The model under review builds one solid part; all positions refer to its coordinate system, in mm. A direction names the side the tool comes from. Coordinates: 2 decimals unless noted, no trailing zeros. Order: outer loops, then holes, each group sorted by start corner. A loop starts at its lowest first (then second) coordinate and runs counter-clockwise, first axis right, second up. Notation, with made-up numbers: (6, -34) - (18, -34) arc R30 ccw to (18, -12) - close; hole circle Ø2 at (73.5, -22). An arc over 180 degrees is marked (long way). Answer in a Markdown table with one row per item.
```python
from build123d import *

# Parameters (mm, degrees)
BOSS_EXTRUDE1_DEPTH = 40
SKETCH3_OUTSIDE_W   = 68.248
SKETCH3_OUTSIDE_H   = 58.248
CUT_EXTRUDE1_DEPTH  = 40
SKETCH4_OUTSIDE_W   = 68.248
SKETCH4_OUTSIDE_H   = 58.248
SKETCH4_OUTSIDE_R   = 10
CUT_EXTRUDE4_DEPTH  = 40


with BuildPart() as part:
    # Sketch2 → Boss-Extrude1 (new body)
    with BuildSketch(Plane.XY):
        with BuildLine():
            Line((2.466960352, 28.854625551), (-27.533039648, 28.854625551))
            Line((-27.533039648, 28.854625551), (-27.533039648, -1.145374449))
            ThreePointArc((-27.533039648, -1.145374449), (-21.675175271, -15.287510073), (-7.533039648, -21.145374449))
            Line((-7.533039648, -21.145374449), (22.466960352, -21.145374449))
            Line((22.466960352, -21.145374449), (22.466960352, -11.145374449))
            Line((22.466960352, -11.145374449), (-7.533039648, -11.145374449))
            ThreePointArc((-7.533039648, -11.145374449), (-14.604107459, -8.216442261), (-17.533039648, -1.145374449))
            Line((-17.533039648, -1.145374449), (-17.533039648, 18.854625551))
            Line((-17.533039648, 18.854625551), (2.466960352, 18.854625551))
            Line((2.466960352, 18.854625551), (2.466960352, 28.854625551))
        make_face()
    extrude(amount=BOSS_EXTRUDE1_DEPTH)

    # Sketch3 outside → Cut-Extrude1 (cut)
    with BuildSketch(Plane(origin=(0, 28.854625551, 0), x_dir=(1, 0, 0), z_dir=(0, 1, 0))):
        with Locations((-2.533, -20)):
            Rectangle(SKETCH3_OUTSIDE_W, SKETCH3_OUTSIDE_H)
        with BuildLine():
            Line((-27.533039648, 0), (-27.533039648, -40))
            Line((-27.533039648, -40), (-7.533039648, -40))
            ThreePointArc((-7.533039648, -40), (-0.461971836, -37.071067812), (2.466960352, -30))
            Line((2.466960352, -30), (2.466960352, -10))
            ThreePointArc((2.466960352, -10), (-0.461971836, -2.928932188), (-7.533039648, 0))
            Line((-7.533039648, 0), (-27.533039648, 0))
        make_face(mode=Mode.SUBTRACT)
    extrude(amount=-CUT_EXTRUDE1_DEPTH, mode=Mode.SUBTRACT)

    # Sketch4 outside → Cut-Extrude4 (cut)
    # profile 1 of 2: a face of its own
    with BuildSketch(Plane.XZ.offset(21.145374449)):
        with Locations((-2.533, 20)):
            Rectangle(SKETCH4_OUTSIDE_W, SKETCH4_OUTSIDE_H)
        with BuildLine():
            Line((-7.533039648, 40), (-27.533039648, 40))
            Line((-27.533039648, 40), (-27.533039648, 0))
            Line((-27.533039648, 0), (-7.533039648, 0))
            Line((-7.533039648, 0), (2.466960352, 0))
            ThreePointArc((2.466960352, 0), (22.466960352, 20), (2.466960352, 40))
            Line((2.466960352, 40), (-7.533039648, 40))
        make_face(mode=Mode.SUBTRACT)
    # profile 2 of 2: a face of its own
    with BuildSketch(Plane.XZ.offset(21.145374449)):
        with Locations(Location((2.466960352, 20, 0), (0, 0, 180))):
            Circle(SKETCH4_OUTSIDE_R)
    extrude(amount=-CUT_EXTRUDE4_DEPTH, mode=Mode.SUBTRACT)


solid = part.part
```
Item 1: We need section A-A, the plane x = 10. Write out the cut boundary in (y, z).
Check values:
| item | result |
|---|---|
| outline | (-21.15, 1.47) - (-11.15, 1.47) - (-11.15, 13.42) - (-21.15, 13.42) - close; (-21.15, 26.58) - (-11.15, 26.58) - (-11.15, 38.53) - (-21.15, 38.53) - close |
Item 2: To check wall thickness, follow line 1 (X direction, y = -13.5, z = 20); line 2 (X direction, y = -19, z = 20); line 3 (X direction, y = 7.5, z = 38). State the ranges of each line that lie inside material, in increasing order. Write a range as from..to.
Check values:
| item | result |
|---|---|
| line 1 | -23.26..-7.53, 12.47..22.47 |
| line 2 | -16.54..-7.53, 12.47..22.47 |
| line 3 | -27.53..-17.53 |
Item 3: Mouldability with a two-part tool opening along Y and no side actions: class faces 5 (the face through (-8, 18.855, 20)), 6 (the face through (-0.54, 23.92, 37.15)), 7 (the face through (-21.83, -15.13, 19.72)) as +Y half, -Y half, draft (parallel to the pull), parting line (faces both ways), or undercut.
Check values:
| item | result |
|---|---|
| face 5 | undercut |
| face 6 | draft |
| face 7 | -Y half |
Item 4: We need section B-B, the plane z = 15.5. Write out the cut boundary in (x, y), then the cut area to 3 significant figures.
Check values:
| item | result |
|---|---|
| outline | (-27.53, -1.15) arc R20 ccw to (-7.53, -21.15) - (-6.46, -21.15) - (-6.46, -11.15) - (-7.53, -11.15) arc R10 cw to (-17.53, -1.15) - (-17.53, 18.85) - (2.47, 18.85) - (2.47, 28.85) - (-27.53, 28.85) - close; (11.4, -21.15) - (21.95, -21.15) - (21.95, -11.15) - (11.4, -11.15) - close |
| area | 852 mm^2 |
Item 5: Clearance check with flat-ended pins moving along their axes: pin 1 Ø4 at (y, z) = (-5, 26) entering from -X; pin 2 Ø8 at (y, z) = (2, 34.5) entering from +X; pin 3 Ø12 at (x, z) = (17.5, 10.5) entering from +Y. State where each tip first meets the part, or that it passes through.
Check values:
| item | result |
|---|---|
| pin 1 | x = -27.45 |
| pin 2 | x = -17.5 |
| pin 3 | y = -11.15 |
Item 6: We need section D-D, the plane z = 7.5. Write out the cut boundary in (x, y), then the cut area to 3 significant figures.
Check values:
| item | result |
|---|---|
| outline | (-27.53, -1.15) arc R20 ccw to (-7.53, -21.15) - (18.08, -21.15) - (18.08, -11.15) - (-7.53, -11.15) arc R10 cw to (-17.53, -1.15) - (-17.53, 18.85) - (2.15, 18.85) - (2.15, 28.85) - (-27.53, 28.85) - close |
| area | 989 mm^2 |
Item 7: We need section C-C, the plane x = -2. Write out the cut boundary in (y, z), then the cut area to 3 significant figures.
Check values:
| item | result |
|---|---|
| outline | (-21.15, 0) - (-11.15, 0) - (-11.15, 11.05) - (-21.15, 11.05) - close; (-21.15, 28.95) - (-11.15, 28.95) - (-11.15, 40) - (-21.15, 40) - close; (18.85, 1.67) - (28.85, 1.67) - (28.85, 38.33) - (18.85, 38.33) - close |
| area | 588 mm^2 |
Item 8: Tool access review of faces 1 (the face through (9.8, -16.2, 13.2)), 2 (the face through (-27.533, 14, 20)), 3 (the face through (-0.38, 23.92, 3.01)), 4 (the face through (-17.533, 9, 20)): name each direction out of +Z, -Z, +X, -X, +Y, -Y from which nothing blocks a thin tool from reaching the whole face with its end or side.
Check values:
| item | result |
|---|---|
| face 1 | -Y |
| face 2 | +Z, -Z, -X, +Y, -Y |
| face 3 | -Z, +X, +Y |
| face 4 | +Z, -Z, +X |
